Verification items for the finished model (mm, model axes). Round coordinates to 2 decimals unless told otherwise and drop trailing zeros. Write each loop counter-clockwise with the first axis right and the second up, starting at its lowest first coordinate (ties: lowest second). Pieces come first, ordered by that corner, then holes. Notation, with made-up numbers: M 75,-23.5 L 128,-23.5 A30 cw 128,6.5 Z; hole C 77.5,7 d6. An arc over 180 degrees is marked long. Answer in a Markdown table with one row per item. Add a question column.
1. Sectioned sample at A-A on z = -72. Record the cut outline in (x, y).
2. Sectioned sample at B-B on x = 46. Record the cut outline in (y, z).
3. Material ranges on probe 1 along Z at (x, y) = (25, 1.7); probe 2 along Z at (x, y) = (225, 1.85); probe 3 along X at (y, z) = (0.65, -25), recorded low to high.
4. Go/stop test with flat-tipped pins: pin 1 Ø1.5 at (x, z) = (189, -37) entering from +Y; pin 2 Ø2.5 at (x, z) = (225, -125) entering from -Y; pin 3 Ø5.5 at (x, z) = (25, -225) entering from +Y; pin 4 Ø4 at (x, z) = (25, -25) entering from +Y. Record where each tip stops, or that it passes through.
```python
from build123d import *

# Parameters (mm, degrees)
SKETCH1_W                                       = 250
SKETCH1_H                                       = 250
BOSS_EXTRUDE2_DEPTH                             = 4.5
CSK_FOR_M3_FLAT_HEAD_MACHINE_SCREW1_D           = 3.4
CSK_FOR_M3_FLAT_HEAD_MACHINE_SCREW1_CSINK_D     = 6.3
CSK_FOR_M3_FLAT_HEAD_MACHINE_SCREW1_CSINK_ANGLE = 90
SKETCH5_W                                       = 100
SKETCH5_H                                       = 100
BOSS_EXTRUDE3_DEPTH                             = 0.1


with BuildPart() as part:
    # Sketch1 → Boss-Extrude2 (new body)
    with BuildSketch(Plane(origin=(0, 0, 0), x_dir=(1, 0, 0), z_dir=(0, 1, 0))):
        with Locations((125, 125)):
            Rectangle(SKETCH1_W, SKETCH1_H)
    extrude(amount=BOSS_EXTRUDE2_DEPTH)

    # CSK for M3 Flat Head Machine Screw1 (through all)
    with Locations(Plane(origin=(0, 4.5, 0), x_dir=(1, 0, 0), z_dir=(0, 1, 0))):
        with Locations((25, 25), (25, 225), (225, 125)):
            CounterSinkHole(CSK_FOR_M3_FLAT_HEAD_MACHINE_SCREW1_D / 2, CSK_FOR_M3_FLAT_HEAD_MACHINE_SCREW1_CSINK_D / 2, counter_sink_angle=CSK_FOR_M3_FLAT_HEAD_MACHINE_SCREW1_CSINK_ANGLE)

    # Sketch5 → Boss-Extrude3 (add)
    with BuildSketch(Plane(origin=(0, 4.5, 0), x_dir=(1, 0, 0), z_dir=(0, 1, 0))):
        with Locations((125, 125)):
            Rectangle(SKETCH5_W, SKETCH5_H)
    extrude(amount=BOSS_EXTRUDE3_DEPTH)


solid = part.part
```
Geometry check:
| question | item | result |
|---|---|---|
| 1 | outline | M 0,0 L 250,0 L 250,4.5 L 0,4.5 Z |
| 2 | outline | M 0,-250 L 4.5,-250 L 4.5,0 L 0,0 Z |
| 3 | probe 1 | z = -250 to -226.7, -223.3 to -26.7, -23.3 to 0 |
| 3 | probe 2 | z = -250 to -126.7, -123.3 to 0 |
| 3 | probe 3 | x = 0 to 23.3, 26.7 to 250 |
| 4 | pin 1 | stops at y = 4.5 |
| 4 | pin 2 | passes through |
| 4 | pin 3 | stops at y = 4.1 |
| 4 | pin 4 | stops at y = 3.35 |
